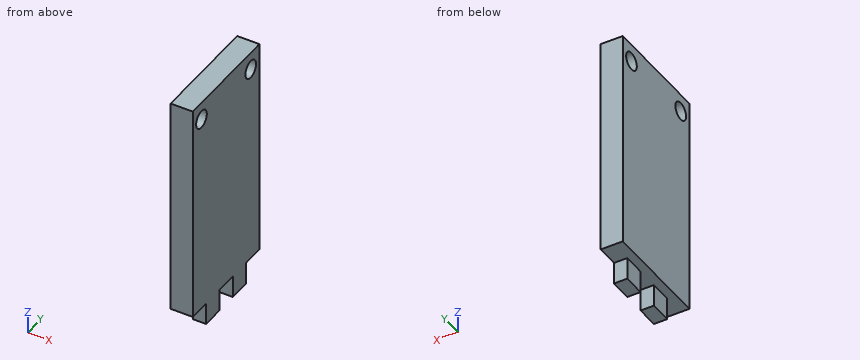
from build123d import *

# Parameters (mm, degrees)
SKETCH1_W           = 5
SKETCH1_H           = 25
BOSS_EXTRUDE1_DEPTH = 50
SKETCH2_R           = 2
CUT_EXTRUDE1_DEPTH  = 15
SKETCH3_W           = 3
SKETCH3_H           = 4.998554169
SKETCH3_H_2         = 5
BOSS_EXTRUDE2_DEPTH = 5


with BuildPart() as part:
    # Sketch1 → Boss-Extrude1 (new body)
    with BuildSketch(Plane.XY):
        with Locations((8.657024793, -1.859504132)):
            Rectangle(SKETCH1_W, SKETCH1_H)
    extrude(amount=BOSS_EXTRUDE1_DEPTH)

    # Sketch2 → Cut-Extrude1 (cut)
    with BuildSketch(Plane.ZY.offset(-6.157024793)):
        with Locations(Location((46, -11.109504132, 0), (0, 0, 270))):
            Circle(SKETCH2_R)
        with Locations(Location((46, 7.390495868, 0), (0, 0, 270))):
            Circle(SKETCH2_R)
    extrude(amount=-CUT_EXTRUDE1_DEPTH, mode=Mode.SUBTRACT)

    # Sketch3 → Boss-Extrude2 (add)
    with BuildSketch(Plane(origin=(0, 0, 0), x_dir=(-1, 0, 0), z_dir=(0, 0, -1))):
        with Locations((-9.657024793, 3.139772953)):
            Rectangle(SKETCH3_W, SKETCH3_H)
        with Locations((-9.657024793, -6.859504132)):
            Rectangle(SKETCH3_W, SKETCH3_H_2)
    extrude(amount=BOSS_EXTRUDE2_DEPTH)


solid = part.part
Geometry: final body of the model. Coordinates: model frame, mm. Round coordinates to 2 decimals unless told otherwise and drop trailing zeros. Order: outer loops, then holes, each group sorted by start corner. A loop starts at its lowest first (then second) coordinate and runs counter-clockwise, first axis right, second up. Notation, with made-up numbers: (74.5, -25.75) - (95.5, -25.75) arc R16 cw to (95.5, -13.75) - close; hole circle Ø4 at (6.25, -33). An arc over 180 degrees is marked (long way). Write each question's results on one line, items separated by ' | '.
Item 1: Section A-A, the plane z = 46. Return the cut outline in (x, y).
Completed:
outline: (6.16, -14.36) - (11.16, -14.36) - (11.16, -13.11) - (6.16, -13.11) - close; (6.16, -9.11) - (11.16, -9.11) - (11.16, 5.39) - (6.16, 5.39) - close; (6.16, 9.39) - (11.16, 9.39) - (11.16, 10.64) - (6.16, 10.64) - close
Item 2: Material intervals for line 1 along Z through (x, y) = (7.4, -11.25); line 2 along Z through (x, y) = (10.05, 8); line 3 along Z through (x, y) = (10.85, 0), sorted ascending. Write a range as [from, to].
Completed:
line 1: [0, 44], [48, 50] | line 2: [0, 44.1], [47.9, 50] | line 3: [0, 50]
Item 3: First-contact query: pin 1 Ø6.5 at (y, z) = (-11.11, 46) entering from +X; pin 2 Ø2.5 at (x, z) = (10, -3) entering from -Y; pin 3 Ø2.5 at (x, z) = (9.5, -2) entering from +Y; pin 4 Ø2.5 at (y, z) = (-8, -2) entering from -X. Flat tips, straight axial feed; report the tip coordinate or a pass-through.
Completed:
pin 1: x = 11.16 | pin 2: y = -9.36 | pin 3: y = 5.64 | pin 4: x = 8.16
Item 4: Section B-B, the plane z = -0.5. Return the cut outline in (x, y).
Completed:
outline: (8.16, -9.36) - (11.16, -9.36) - (11.16, -4.36) - (8.16, -4.36) - close; (8.16, 0.64) - (11.16, 0.64) - (11.16, 5.64) - (8.16, 5.64) - close
Item 5: Section C-C, the plane x = 9.4. Return the cut outline in (y, z), and give its area (3 significant figures).
Completed:
outline: (-14.36, 0) - (-9.36, 0) - (-9.36, -5) - (-4.36, -5) - (-4.36, 0) - (0.64, 0) - (0.64, -5) - (5.64, -5) - (5.64, 0) - (10.64, 0) - (10.64, 50) - (-14.36, 50) - close; hole circle Ø4 at (-11.11, 46); hole circle Ø4 at (7.39, 46) | area: 1,270 mm^2
Item 6: Section D-D, the plane y = 0. Return the cut outline in (x, z), and give its area (3 significant figures).
Completed:
outline: (6.16, 0) - (11.16, 0) - (11.16, 50) - (6.16, 50) - close | area: 250 mm^2
